Input: part model. Units: mm. Frame: model coordinates. Give positions to 0.01 mm unless a question says otherwise; leave off trailing zeros. Write each loop counter-clockwise with the first axis right and the second up, starting at its lowest first coordinate (ties: lowest second). Pieces come first, ordered by that corner, then holes. Notation, with made-up numbers: (-12.5, -35) - (45.5, -35) arc R15 ccw to (45.5, -22) - close; hole circle Ø7 at (-11, 68). An arc over 180 degrees is marked (long way). Answer as CSV lines item,"result".
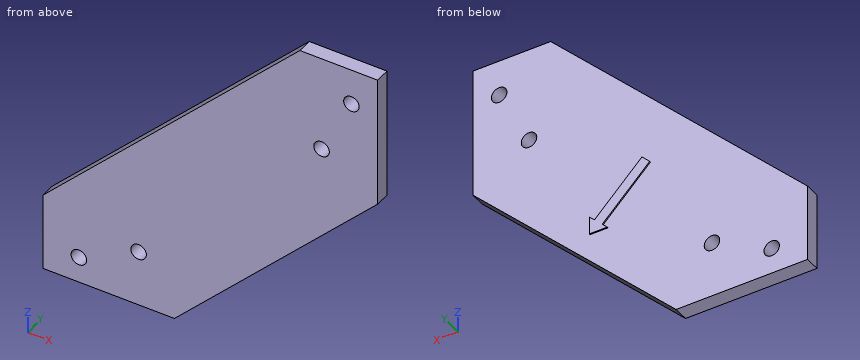
```python
from build123d import *

# Parameters (mm, degrees)
SKETCH1_R           = 1.651
BOSS_EXTRUDE2_DEPTH = 3.175
BOSS_EXTRUDE3_DEPTH = 0.254


with BuildPart() as part:
    # Sketch1 → Boss-Extrude2 (new body)
    with BuildSketch(Plane(origin=(0, 0, 0), x_dir=(1, 0, 0), z_dir=(0, 1, 0))):
        Polygon((0, -43.18), (-43.18, 0), (-71.12, 0), (-71.12, -16.51), (-16.51, -71.12), (0, -71.12), align=None)
        with Locations((-5.55605696, -63.5)):
            Circle(SKETCH1_R, mode=Mode.SUBTRACT)
        with Locations((-11.905836488, -50.8)):
            Circle(SKETCH1_R, mode=Mode.SUBTRACT)
        with Locations((-63.5, -5.55605696)):
            Circle(SKETCH1_R, mode=Mode.SUBTRACT)
        with Locations((-50.8, -11.905836488)):
            Circle(SKETCH1_R, mode=Mode.SUBTRACT)
    extrude(amount=BOSS_EXTRUDE2_DEPTH)

    # Sketch5 → Boss-Extrude3 (add)
    with BuildSketch(Plane(origin=(0, 3.175, 0), x_dir=(1, 0, 0), z_dir=(0, 1, 0))):
        Polygon((-24.899422015, -24.239032228), (-28.709422015, -24.239032228), (-27.63179128, -25.316662963), (-37.727112803, -35.411984485), (-36.072374272, -37.066723016), (-25.977052749, -26.971401493), (-24.899422015, -28.049032228), align=None)
    extrude(amount=BOSS_EXTRUDE3_DEPTH)


solid = part.part
```
Item 1: Contact query for flat-ended pins moving along their axis: pin 1 (2 mm diameter, centred on x = -45.5, y = 3, fed in from +Z); pin 2 (5.5 mm diameter, centred on x = -63.5, z = 5.56, fed in from +Y) (3 decimals); pin 3 (1.5 mm diameter, centred on y = 3, z = 39, fed in from +X); pin 4 (2 mm diameter, centred on x = -5.56, z = 63.5, fed in from -Y). Output: stop coordinate, or through.
The answers:
pin 1,"z = 43.13"
pin 2,"y = 3.175"
pin 3,"x = -3.43"
pin 4,"through"
Item 2: Cut plane B-B on z = 63.5. Return the cut outline in (x, y) (3 decimals).
The answers:
outline,"(-24.13, 0) - (-7.207, 0) - (-7.207, 3.175) - (-24.13, 3.175) - close; (-3.905, 0) - (0, 0) - (0, 3.175) - (-3.905, 3.175) - close"
Item 3: Cut plane C-C on y = 1. Return the cut outline in (x, z).
The answers:
outline,"(-71.12, 0) - (-43.18, 0) - (0, 43.18) - (0, 71.12) - (-16.51, 71.12) - (-71.12, 16.51) - close; hole circle Ø3.3 at (-63.5, 5.56); hole circle Ø3.3 at (-50.8, 11.91); hole circle Ø3.3 at (-11.91, 50.8); hole circle Ø3.3 at (-5.56, 63.5)"
Item 4: Cut plane D-D on x = -41. Return the cut outline in (y, z) (3 decimals).
The answers:
outline,"(0, 2.18) - (3.175, 2.18) - (3.175, 46.63) - (0, 46.63) - close"
Item 5: Ray query, line 1 (Z direction, x = -11.5, y = 2.55); line 2 (Z direction, x = -63.5, y = 1.3); line 3 (Y direction, x = -37, z = 48.5) (3 decimals). Return the intervals inside material, ascending. Write a range as from..to.
The answers:
line 1,"31.68..49.2, 52.4..71.12"
line 2,"0..3.91, 7.21..24.13"
line 3,"0..3.175"
Item 6: Cut plane A-A on x = -50.8. Return the cut outline in (y, z) (3 decimals), plus the area to 3 significant figures.
The answers:
outline,"(0, 0) - (3.175, 0) - (3.175, 10.255) - (0, 10.255) - close; (0, 13.557) - (3.175, 13.557) - (3.175, 36.83) - (0, 36.83) - close"
area,"106 mm²"
